```python
from build123d import *


with BuildPart() as part:
    # Esquisse1 → Révolution1 (revolve)
    with BuildSketch(Plane.XY, mode=Mode.PRIVATE) as r_volution1_sk:
        Polygon((42, 3), (72, 3), (72, 2), (79, 2), (79, 0), (0, 0), (0, 2), (7, 2), (7, 3), (30, 3), (30, 4), (42, 4), align=None)
    revolve(r_volution1_sk.sketch.rotate(Axis((0, 0, 0), (1, 0, 0)), 90), axis=Axis((0, 0, 0), (1, 0, 0)))  # turned: the seam where the file's is


solid = part.part
```
Input: part model. Units: mm. Frame: model coordinates. A direction names the side the tool comes from. Give positions to 0.01 mm unless a question says otherwise; leave off trailing zeros. Order: outer loops, then holes, each group sorted by start corner. A loop starts at its lowest first (then second) coordinate and runs counter-clockwise, first axis right, second up.
1. Section A-A on y = 0. Return the cut outline in (x, z).
Derived:
outline: (0, -2) - (7, -2) - (7, -3) - (30, -3) - (30, -4) - (42, -4) - (42, -3) - (72, -3) - (72, -2) - (79, -2) - (79, 2) - (72, 2) - (72, 3) - (42, 3) - (42, 4) - (30, 4) - (30, 3) - (7, 3) - (7, 2) - (0, 2) - close
2. Pin query (flat end, axial travel): pin 1 (1.5 mm diameter, centred on x = 26, z = -3, fed in from -Y). Return the tip coordinate at first contact, or that it passes through.
Derived:
pin 1: stops at y = -1.98
3. Reachability of faces 1 (the flat face through (42, -3, 1)), 2 (the flat face through (79, 0, 0)), 3 (the cylindrical face through (18.66, -0.9, 2.86)) from +Z, -Z, +X, -X, +Y, -Y: full face, straight path, thin tool, end or side. Return the list, or none.
Derived:
face 1: +X
face 2: +Z, -Z, +X, +Y, -Y
face 3: -X
4. Material intervals for L1, parallel to X at y = -3, z = -2.5; L2, parallel to X at y = 0, z = -2.25; L3, parallel to Z at x = 28, y = 0.25, sorted ascending.
Derived:
L1: x = 30 to 42
L2: x = 7 to 72
L3: z = -2.99 to 2.99
5. Section C-C on x = 49. Return the cut outline in (y, z), and give its area (3 significant figures).
Derived:
outline: circle Ø6 at (0, 0)
area: 28.3 mm2
